from build123d import *

# Parameters (mm, degrees)
BOSS_EXTRUDE1_DEPTH = 10
SKETCH4_R           = 2.452335066
CUT_EXTRUDE2_DEPTH  = 2
SKETCH4_2_R         = 2.452335066
CUT_EXTRUDE3_DEPTH  = 34.35416016
FILLET2_R           = 1


with BuildPart() as part:
    # Sketch2 → Boss-Extrude1 (new body)
    with BuildSketch(Plane(origin=(0, 0, 0), x_dir=(1, 0, 0), z_dir=(0, 1, 0))):
        with BuildLine():
            Line((-13, 15), (-13, 16.317168872))
            ThreePointArc((-13, 16.317168872), (-13.582365465, 17.22578397), (-14.651162791, 17.076106959))
            ThreePointArc((-14.651162791, 17.076106959), (0, -22.5), (14.651162791, 17.076106959))
            ThreePointArc((14.651162791, 17.076106959), (13.582365465, 17.22578397), (13, 16.317168872))
            Line((13, 16.317168872), (13, 15))
            ThreePointArc((13, 15), (0, 2), (-13, 15))
        make_face()
    extrude(amount=BOSS_EXTRUDE1_DEPTH)

    # Sketch4 → Cut-Extrude2 (cut)
    with BuildSketch(Plane(origin=(0, 10, 0), x_dir=(1, 0, 0), z_dir=(0, 1, 0))):
        with BuildLine():
            Line((-14.9, -3.5), (0, -2))
            Line((0, -2), (14.9, -3.5))
            ThreePointArc((14.9, -3.5), (17.4, -6), (14.9, -8.5))
            Line((14.9, -8.5), (0, -10))
            Line((0, -10), (-14.9, -8.5))
            ThreePointArc((-14.9, -8.5), (-17.4, -6), (-14.9, -3.5))
        make_face()
        with Locations(Location((0, -6, 0), (0, 0, 270))):
            Circle(SKETCH4_R, mode=Mode.SUBTRACT)
    extrude(amount=-CUT_EXTRUDE2_DEPTH, mode=Mode.SUBTRACT)

    # Sketch4_2 → Cut-Extrude3 (cut, through all)
    with BuildSketch(Plane(origin=(0, 10, 0), x_dir=(1, 0, 0), z_dir=(0, 1, 0))):
        with Locations(Location((0, -6, 0), (0, 0, 270))):
            Circle(SKETCH4_2_R)
    extrude(amount=-CUT_EXTRUDE3_DEPTH, mode=Mode.SUBTRACT)

    # Fillet2
    fillet2_edges = [part.edges().sort_by_distance(p)[0] for p in [
        (0, 10, -2),
        (-13, 10, -15.658584436),
        (-13.582365465, 10, -17.22578397),
        (0, 10, 22.5),
        (13.582365465, 10, -17.22578397),
        (0, 0, 22.5),
        (-13.582365465, 0, -17.22578397),
        (-13, 0, -15.658584436),
        (0, 0, -2),
        (13, 0, -15.658584436),
        (13.582365465, 0, -17.22578397),
        (13, 10, -15.658584436),
    ]]
    fillet(fillet2_edges, radius=FILLET2_R)


solid = part.part
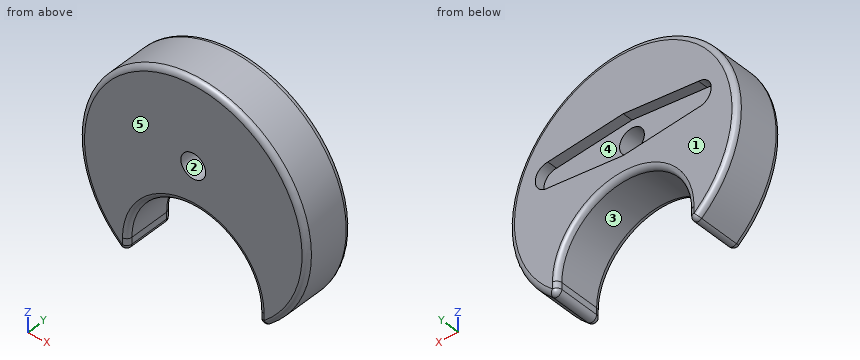
Input: part model. Units: mm. Frame: model coordinates. Face numbers are marked on the shaded views. A direction names the side the tool comes from. Give positions to 0.01 mm unless a question says otherwise; leave off trailing zeros. Order: outer loops, then holes, each group sorted by start corner. A loop starts at its lowest first (then second) coordinate and runs counter-clockwise, first axis right, second up. Notation, with made-up numbers: M -6.5,8 L 25.5,8 A13 cw 25.5,16 Z; hole C 50.5,85 d6. An arc over 180 degrees is marked long. Answer as a JSON object with one key per item and string values.
1. Reachability of the marked faces 4 and 5 from +Z, -Z, +X, -X, +Y, -Y: full face, straight path, thin tool, end or side. Return the list, or none.
Result sheet:
{"face 4": "+Y", "face 5": "+Z, -Z, +X, -X, -Y"}
2. Pull-direction query (Z, two-part tool) for the marked faces 1, 2 and 3; classes: +Z half, -Z half, draft (parallel to the pull), parting line (faces both ways), or undercut.
Result sheet:
{"face 1": "draft", "face 2": "undercut", "face 3": "-Z half"}
3. First-contact query: P1, Ø1.4, axis at y = 4, z = -15.5, coming from the -X side; P2, Ø1, axis at y = 6.5, z = 2, coming from the +X side; P3, Ø5, axis at x = 8, y = 1, coming from the -Z side. Flat tips, straight axial feed; report the tip coordinate or a pass-through.
Result sheet:
{"P1": "x = -16.95", "P2": "x = 22.45", "P3": "z = -7.34"}
4. Ray query, line 1 (Y direction, x = 11.5, z = 5); line 2 (X direction, y = 4, z = 6); line 3 (X direction, y = 7.75, z = -10). Return the intervals inside material, ascending. Write a range as [from, to].
Result sheet:
{"line 1": "[0, 8]", "line 2": "[-21.69, -2.45], [2.45, 21.69]", "line 3": "[-20.16, -12], [12, 20.16]"}
5. Cut plane A-A, the plane y = 3.25. Output: boundary loops of the cut face in (x, z), and give its area (3 significant figures).
Result sheet:
{"outline": "M -14.65,-17.08 A1 ccw -13,-16.32 L -13,-15 A13 cw 13,-15 L 13,-16.32 A1 ccw 14.65,-17.08 A22.5 ccw long Z; hole C 0,6 d4.9", "area": "1,140 mm²"}
